```python
from build123d import *

# Parameters (mm, degrees)
BOSS_EXTRUDE1_DEPTH         = 1.5875
F_6_CLEARANCE_HOLE2_D       = 3.6576
F_6_CLEARANCE_HOLE2_DEPTH   = 38.354
F_6_CLEARANCE_HOLE2_TIP     = 1.0988539
SKETCHED_START              = -6.35
SKETCHED_BEND10_DEPTH       = 12.7
SKETCHED_BEND10_2_DEPTH     = 12.7
CUT_EXTRUDE1_DEPTH          = 45.703347893
F_1_4_CLEARANCE_HOLE1_D     = 6.5278
F_1_4_CLEARANCE_HOLE1_DEPTH = 38.354
F_1_4_CLEARANCE_HOLE1_TIP   = 1.961148974


# Read off the part's stored shape, not the designer's step: Sketched Bend10
with BuildPart() as part:
    # Sketch1 → Boss-Extrude1 (new body)
    with BuildSketch(Plane.XY):
        Polygon((-17.78, -25.4), (17.78, -25.4), (17.78, 25.4), (6.35, 25.4), (6.35, 43.18), (-6.35, 43.18), (-6.35, 25.4), (-17.78, 25.4), align=None)
    extrude(amount=BOSS_EXTRUDE1_DEPTH)

    # #6 Clearance Hole2
    with Locations(Plane(origin=(0, 0, 0), x_dir=(-1, 0, 0), z_dir=(0, 0, -1))):
        with Locations((0, 9.5), (0, -9.5)):
            Hole(F_6_CLEARANCE_HOLE2_D / 2, depth=F_6_CLEARANCE_HOLE2_DEPTH)
            with Locations((0, 0, -(F_6_CLEARANCE_HOLE2_DEPTH + F_6_CLEARANCE_HOLE2_TIP / 2))):  # 118° drill point
                Cone(0, F_6_CLEARANCE_HOLE2_D / 2, F_6_CLEARANCE_HOLE2_TIP, mode=Mode.SUBTRACT)

    # Sketched Bend10 outline → Sketched Bend10 (cut)
    with BuildSketch(Plane.YZ.offset(SKETCHED_START)):
        with BuildLine():
            ThreePointArc((25.769655935, 1.5875), (28.279713828, 1.180173678), (30.532155935, 0))
            Line((30.532155935, 0), (43.18, 0))
            Line((43.18, 0), (43.18, 1.5875))
            Line((43.18, 1.5875), (25.769655935, 1.5875))
        make_face()
    extrude(amount=SKETCHED_BEND10_DEPTH, mode=Mode.SUBTRACT)

    # Sketched Bend10 2 outline → Sketched Bend10 2 (add)
    with BuildSketch(Plane.YZ.offset(SKETCHED_START)):
        with BuildLine():
            Line((39.725932738, -9.080956652), (31.382316011, -0.737339924))
            ThreePointArc((31.382316011, -0.737339924), (30.970319757, -0.353584232), (30.532155935, 0))
            Line((30.532155935, 0), (25.769655935, 0))
            ThreePointArc((25.769655935, 0), (28.19969573, -0.483364969), (30.259783996, -1.859871939))
            Line((30.259783996, -1.859871939), (38.603400723, -10.203488667))
            Line((38.603400723, -10.203488667), (39.725932738, -9.080956652))
        make_face()
    extrude(amount=SKETCHED_BEND10_2_DEPTH)

    # Sketch18 → Cut-Extrude1 (cut, through all)
    with BuildSketch(Plane(origin=(0, 0, 0), x_dir=(-1, 0, 0), z_dir=(0, 0, -1))):
        with BuildLine():
            Line((-17.78, -25.4), (0, -25.4))
            ThreePointArc((0, -25.4), (-9.602697629, -23.51485059), (-17.78, -18.139228208))
            Line((-17.78, -18.139228208), (-17.78, -25.4))
        make_face()
        with BuildLine():
            Line((17.78, -25.4), (17.78, -18.139228208))
            ThreePointArc((17.78, -18.139228208), (9.602697629, -23.51485059), (0, -25.4))
            Line((0, -25.4), (17.78, -25.4))
        make_face()
    extrude(amount=-CUT_EXTRUDE1_DEPTH, mode=Mode.SUBTRACT)

    # 1/4 Clearance Hole1
    with Locations(Plane(origin=(0, 15.322488043, 15.322488043), x_dir=(1, 0, 0), z_dir=(0, 0.7071067811865487, 0.7071067811865465))):
        with Locations((0, 27.173236583)):
            Hole(F_1_4_CLEARANCE_HOLE1_D / 2, depth=F_1_4_CLEARANCE_HOLE1_DEPTH)
            with Locations((0, 0, -(F_1_4_CLEARANCE_HOLE1_DEPTH + F_1_4_CLEARANCE_HOLE1_TIP / 2))):  # 118° drill point
                Cone(0, F_1_4_CLEARANCE_HOLE1_D / 2, F_1_4_CLEARANCE_HOLE1_TIP, mode=Mode.SUBTRACT)


solid = part.part
```
Geometry: final body of the model. Coordinates: model frame, mm. A direction names the side the tool comes from. Give positions to 0.01 mm unless a question says otherwise; leave off trailing zeros. Loops run counter-clockwise (first coordinate to the right, second up) from the corner with the lowest first, then second, coordinate; pieces in that order, holes last. Notation, with made-up numbers: (12, -18.5) - (45, -18.5) arc R6 ccw to (45, -14.5) - close; hole circle Ø2 at (75, 41.25). An arc over 180 degrees is marked (long way). Answer as CSV lines item,"result". Start each with the question number.
(1) Pin query (flat end, axial travel): P1, Ø2, axis at x = 6, y = -18.5, coming from the -Z side; P2, Ø3, axis at x = 4, y = 30.5, coming from the +Z side; P3, Ø1.3, axis at x = -10.5, z = 0.5, coming from the +Y side. Return the tip coordinate at first contact, or that it passes through.
(2) Ray query, line 1 along Z through (x, y) = (2, -16); line 2 along Z through (x, y) = (2, 31); line 3 along Y through (x, z) = (6, -5.25). Return the intervals inside material, ascending. Write a range as [from, to].
(3) Reachability of faces 1 (the face through (2.406, 35.528, -6.021)), 2 (the face through (6.35, 33, -3)), 3 (the face through (-6.35, 33, -3)) from +Z, -Z, +X, -X, +Y, -Y: full face, straight path, thin tool, end or side. Return the list, or none.
(4) Section query C-C (x = -14). Output: boundary loops of the cut face in (y, z), and give its area (3 significant figures).
(5) Section query B-B (y = 15.5). Output: boundary loops of the cut face in (x, z).
(6) Section query A-A (y = -9.5). Output: boundary loops of the cut face in (x, z), and give its area (3 significant figures).
(7) Mould query, pull axis Y, two halves, no side actions, for faces 4 (the face through (0, 1, 0)), 5 (the face through (-0.09, 28.17, -0.47)), 6 (the face through (-0.089, 37.467, -6.822)), 7 (the face through (-1.451, 8.387, 0.805)). Classes: +Y half, -Y half, draft (parallel to the pull), parting line (faces both ways), or undercut.
Worked answers:
1,P1,"stops at z = 0"
1,P2,"stops at z = 0.9"
1,P3,"stops at y = 25.4"
2,line 1,"z = [0, 1.59]"
2,line 2,"z = [-2.6, -0.38]"
2,line 3,"y = [33.65, 35.89]"
3,face 1,"none"
3,face 2,"+Z, -Z, +X, +Y"
3,face 3,"+Z, -Z, -X, +Y"
4,outline,"(-21.19, 0) - (25.4, 0) - (25.4, 1.59) - (-21.19, 1.59) - close"
4,area,"74.0 mm^2"
5,outline,"(-17.78, 0) - (17.78, 0) - (17.78, 1.59) - (-17.78, 1.59) - close"
6,outline,"(-17.78, 0) - (-1.83, 0) - (-1.83, 1.59) - (-17.78, 1.59) - close; (1.83, 0) - (17.78, 0) - (17.78, 1.59) - (1.83, 1.59) - close"
6,area,"50.6 mm^2"
7,face 4,"draft"
7,face 5,"-Y half"
7,face 6,"+Y half"
7,face 7,"undercut"
